Autodesk Inventor part; units mm, degrees
ref_plane "YZ Plane" through (0, 0, 0) normal (1, 0, 0) x (0, 1, 0)
ref_plane "XZ Plane" through (0, 0, 0) normal (0, 1, 0) x (-1, 0, 0)
ref_plane "XY Plane" through (0, 0, 0) normal (0, 0, 1) x (1, 0, 0)
sketch "スケッチ1" plane through (0, 0, 0) normal (0, 0, 1) x (1, 0, 0)
  line L0 (0, 0) -> (10, 0)
  line L1 (10, 0) -> (10, 15)
  line L2 (10, 15) -> (0, 15)
  line L3 (0, 15) -> (0, 0)
  circle A0 centre (5, 15) radius 10
  circle A1 centre (5, 15) radius 15
  line L4 (-8.7477, 9) -> (18.7477, 9)
  line L5 (18.7477, 9) -> (18.7477, 21)
  line L6 (18.7477, 21) -> (-8.7477, 21)
  line L7 (-8.7477, 21) -> (-8.7477, 9)
  line L8 (-8.7477, 9) -> (18.7477, 21) construction
  line L9 (18.7477, 9) -> (-8.7477, 21) construction
  point P0 (0, 6.3397)
  point P1 (10, 6.3397)
  point P2 (-8.7477, 9)
  point P3 (-3, 9)
  point P4 (-3, 21)
  point P5 (-8.7477, 21)
  point P6 (13, 21)
  point P7 (13, 9)
  point P8 (18.7477, 9)
  point P9 (10, 9)
  point P10 (0, 9)
  point P11 (-8.7477, 9)
  point P12 (-8.7477, 21)
  point P13 (18.7477, 9)
  point P14 (10, 0.8579)
  point P15 (0, 0.8579)
  point P16 (5, 0)
  dimension "d41" = 30
  dimension "d0" = 15
  dimension "d1" = 20
  dimension "d27" = 10
  dimension "d28" = 5
  dimension "d42" = 12
extrude "押し出し1" add sketch "スケッチ1" along normal blind 10 contours L3 A1 L0 | A1 L1 L0 | A1 L3 A0 L1 | A0 L4 L3 | L3 L4 L1 A0 | L7 L6 A0 L4 | A1 L7 | L1 L4 A0 | L5 A1 | L4 A0 L6 L5 | L4 A0 L6 L1 L2 L3 | L3 L2 L1 L4 | A0 L6
sketch "スケッチ2" plane through (0, 0, 10) normal (0, 0, 1) x (1, 0, 0)
  arc A0 (10, 6.3397) -> (0, 6.3397) centre (5, 15) ccw
  point P0 (0, 0)
  point P1 (5, 15)
hole "穴1" at (5, 15, 10) direction (0, 0, -1) diameter 10.4 end through all
sketch "スケッチ3" plane through (0, 0, 10) normal (0, 0, 1) x (1, 0, 0)
  line L0 (0, 0) -> (10, 0)
  line L1 (4.5, 0) -> (5.5, 0)
  line L2 (5.5, 0) -> (5.5, 15)
  line L3 (5.5, 15) -> (4.5, 15)
  line L4 (4.5, 15) -> (4.5, 0)
  line L5 (0, 6.3397) -> (0, 0)
  circle A0 centre (5, 15) radius 5.2
  point P0 (5, 0)
  point P1 (5, 0)
  dimension "d14" = 1
extrude "押し出し2" cut sketch "スケッチ3" against normal up to surface (10 mm away) contours L4 A0 L2 L0 | L4 L3 L2 A0 picked at (5.0556, 13.2676)
sketch "スケッチ4" plane through (10, 0, 0) normal (1, 0, 0) x (0, 0, -1)
  circle A0 centre (-5, 4) radius 1.5
  line L0 (0, 0) -> (-10, 0)
  line L1 (0, 0) -> (0, 6.3397)
  line L2 (-5, 0) -> (-5, 10)
  point P0 (0, 10)
  dimension "d17" = 4
  dimension "d19" = 3
hole "穴2" at (10, 4, 5) direction (-1, 0, 0) diameter 4.4 end through all
sketch "スケッチ7" plane through (10, 0, 0) normal (1, 0, 0) x (0, 0, -1)
  circle A0 centre (-5, 4) radius 2.2
  line L0 (-5, 8.1569) -> (-1.4, 6.0785)
  line L1 (-1.4, 6.0785) -> (-1.4, 1.9215)
  line L2 (-1.4, 1.9215) -> (-5, -0.1569)
  line L3 (-5, -0.1569) -> (-8.6, 1.9215)
  line L4 (-8.6, 1.9215) -> (-8.6, 6.0785)
  line L5 (-8.6, 6.0785) -> (-5, 8.1569)
  line L6 (-10, 9.8241) -> (-10, 0)
  line L7 (0, 0) -> (0, 6.3397)
  line L8 (-10, 9.8241) -> (0, 9.8241)
  line L9 (0, 9.8241) -> (0, 3.1699)
  line L10 (0, 3.1699) -> (-10, 3.1699)
  line L11 (-10, 3.1699) -> (-10, 9.8241)
  point P0 (-1.4, 3.1699)
  point P1 (0, 6.3397)
  point P2 (-8.6, 3.1699)
  point P3 (-7.0374, 3.1699)
  point P4 (-2.9626, 3.1699)
  dimension "d35" = 7.2
extrude "押し出し5" add sketch "スケッチ7" along normal blind 2 contours L10 L6 L8 L9 L7 L1 L0 L5 L4
chamfer "面取り1" distance 2 angle 45 2 edges at (10, 3.1699, 9.3) (10, 3.1699, 0.7)
sketch "スケッチ8" plane through (0, 0, 0) normal (0, 0, -1) x (-1, 0, 0)
  circle A0 centre (-5, 15) radius 10 construction
  arc A1 (-4.5, 9.8241) -> (-5.5, 9.8241) centre (-5, 15) ccw construction
  point P0 (0, 0)
  point P1 (5, 15)
  point P2 (-15, 15)
  dimension "d44" = 20
hole "穴3" at (-5, 15, 0) at (15, 15, 0) direction (0, 0, 1) diameter 3.4 end through all counterbore diameter 5.9 counterbore depth 3
extrude "押し出し7" cut sketch "スケッチ7" along normal through all contours A0 L10 L4 L5 L0 L1
sketch "スケッチ10" plane through (0, 6.3397, 0) normal (-1, 0, 0) x (0, 0, 1)
  circle A0 centre (5, -2.3397) radius 2.2
  circle A1 centre (5, -2.3397) radius 3.7
  point P0 (0, -6.3397)
  dimension "d57" = 7.4
extrude "押し出し8" cut sketch "スケッチ10" along normal blind 10
hole "穴4" at (10, 6.0785, 8.6) at (10, 6.0785, 1.4) at (10, 8.1569, 5) direction (1, 0, 0) diameter 0.3 end through all
equation "\"d28\" = 0.5 * d27"
properties part number "軸止め" material "ABS プラスチック"
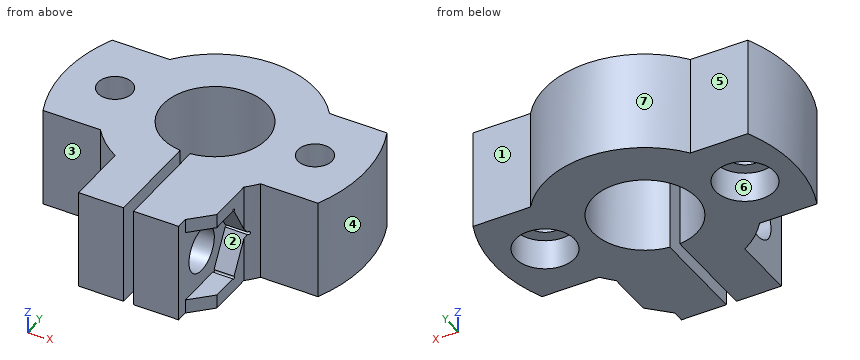
Input: part model. Units: mm. Frame: model coordinates. Face numbers are marked on the shaded views. A direction names the side the tool comes from. Coordinates: 2 decimals unless noted, no trailing zeros. Write each loop counter-clockwise with the first axis right and the second up, starting at its lowest first coordinate (ties: lowest second). Pieces come first, ordered by that corner, then holes. Notation, with made-up numbers: (13.25, -18.75) - (57.25, -18.75) arc R24 cw to (57.25, 12.25) - close; hole circle Ø6 at (4.25, 44). An arc over 180 degrees is marked (long way). Put each result on its own line as item: value. Start each with the question number.
1) Cut plane D-D (z = 6.25). State how many separate pieces and enclosed holes the cut face has, plus the area to 3 significant figures.
2) Contact query for flat-ended pins moving along their axis: pin 1 (3.5 mm diameter, centred on y = 5.5, z = 1, fed in from +X); pin 2 (4.5 mm diameter, centred on x = 14.5, y = 15, fed in from -Z); pin 3 (3 mm diameter, centred on y = 17.5, z = 2.5, fed in from -X). Output: stop coordinate, or through.
3) Reachability of the marked faces 1, 2 and 3 from +Z, -Z, +X, -X, +Y, -Y: full face, straight path, thin tool, end or side. Return the list, or none.
4) Mould query, pull axis X, two halves, no side actions, for the marked faces 4, 5, 6 and 7. Classes: pulls with the +X half, pulls with the -X half, needs draft (parallel to the pull), parting line crosses it, or undercut.
5) Cut plane C-C (x = 15). Return the cut outline in (y, z).
6) Cut plane A-A (y = 15). Return the cut outline in (x, z), plus the area to 3 significant figures.
7) Cut plane B-B (x = 9). Return the cut outline in (y, z), plus the area to 3 significant figures.
8) Ray query, L1, parallel to X at y = 15, z = 7; L2, parallel to Y at x = 8.4, z = 5; L3, parallel to Y at x = 6.75, z = 5.5. Return the intervals inside material, ascending.
Resolved:
1. separate pieces: 3
1. enclosed holes: 2
1. area: 347 mm2
2. pin 1: stops at x = 12
2. pin 2: stops at z = 3
2. pin 3: stops at x = -9.97
3. face 1: +Z, -Z, +X, +Y
3. face 2: +X, -Y
3. face 3: +Z, -Z, -X, -Y
4. face 4: pulls with the +X half
4. face 5: needs draft
4. face 6: undercut
4. face 7: parting line crosses it
5. outline: (9, 0) - (12.05, 0) - (12.05, 3) - (13.3, 3) - (13.3, 10) - (9, 10) - close; (16.7, 3) - (17.95, 3) - (17.95, 0) - (21, 0) - (21, 10) - (16.7, 10) - close
6. outline: (-10, 0) - (-7.95, 0) - (-7.95, 3) - (-6.7, 3) - (-6.7, 10) - (-10, 10) - close; (-3.3, 3) - (-2.05, 3) - (-2.05, 0) - (-0.2, 0) - (-0.2, 10) - (-3.3, 10) - close; (10.2, 0) - (12.05, 0) - (12.05, 3) - (13.3, 3) - (13.3, 10) - (10.2, 10) - close; (16.7, 3) - (17.95, 3) - (17.95, 0) - (20, 0) - (20, 10) - (16.7, 10) - close
6. area: 113 mm2
7. outline: (0, 0) - (11.68, 0) - (11.68, 10) - (0, 10) - close; (18.32, 0) - (24.17, 0) - (24.17, 10) - (18.32, 10) - close; hole circle Ø4.4 at (4, 5)
7. area: 160 mm2
8. L1: x = -10 to -6.7, -3.3 to -0.2, 10.2 to 13.3, 16.7 to 20
8. L2: y = 0 to 1.8, 6.2 to 11.07, 18.93 to 24.4
8. L3: y = 0 to 1.86, 6.14 to 10.1, 19.9 to 24.85
